```python
from build123d import *

# Parameters (mm, degrees)
EXTRUDE_1_DEPTH     = 17.6
FILLET_2_R          = 2
FILLET_3_R          = 8
SKETCH_2_R          = 10
CUT_EXTRUDE_1_DEPTH = 2


with BuildPart() as part:
    # 草圖1 → 填料-伸長1 (new body)
    with BuildSketch(Plane(origin=(0, 0, 0), x_dir=(1, 0, 0), z_dir=(0, 1, 0))):
        with BuildLine():
            Line((-20.05, 15.65), (20.05, 15.65))
            ThreePointArc((20.05, 15.65), (35.7, 0), (20.05, -15.65))
            Line((20.05, -15.65), (-20.05, -15.65))
            ThreePointArc((-20.05, -15.65), (-35.7, 0), (-20.05, 15.65))
        make_face()
    extrude(amount=EXTRUDE_1_DEPTH)

    # 圓角2
    fillet_2_edges = [part.edges().sort_by_distance(p)[0] for p in [
        (35.7, 17.6, 0),
        (0, 17.6, -15.65),
        (-35.7, 17.6, 0),
        (0, 17.6, 15.65),
    ]]
    fillet(fillet_2_edges, radius=FILLET_2_R)

    # 圓角3
    fillet_3_edges = [part.edges().sort_by_distance(p)[0] for p in [
        (0, 0, -15.65),
        (35.7, 0, 0),
        (0, 0, 15.65),
        (-35.7, 0, 0),
    ]]
    fillet(fillet_3_edges, radius=FILLET_3_R)

    # 草圖2 → 除料-伸長1 (cut)
    with BuildSketch(Plane(origin=(0, 17.6, 0), x_dir=(1, 0, 0), z_dir=(0, 1, 0))):
        with Locations(Location((-11.455400627, 0, 0), (0, 0, 270))):
            Circle(SKETCH_2_R)
    extrude(amount=-CUT_EXTRUDE_1_DEPTH, mode=Mode.SUBTRACT)


solid = part.part
```
Geometry check sheet. Reference: the model listing, model coordinates, mm. Round coordinates to 2 decimals unless told otherwise and drop trailing zeros. Order: outer loops, then holes, each group sorted by start corner. A loop starts at its lowest first (then second) coordinate and runs counter-clockwise, first axis right, second up. Notation, with made-up numbers: M 65.5,-12.5 L 115.5,-12.5 A20 ccw 115.5,2.5 Z; hole C -30,-9.75 d10. An arc over 180 degrees is marked long. Write item = value, one per line.
Q1. Section check A-A (x = 11.5). Enter the section's corners in (y, z).
Answer block:
outline = M 0,-7.65 A8 ccw 8,-15.65 L 15.6,-15.65 A2 ccw 17.6,-13.65 L 17.6,13.65 A2 ccw 15.6,15.65 L 8,15.65 A8 ccw 0,7.65 Z
Q2. Section check C-C (x = -9). Enter the section's corners in (y, z), plus the area to 3 significant figures.
Answer block:
outline = M 0,-7.65 A8 ccw 8,-15.65 L 15.6,-15.65 A2 ccw 17.6,-13.65 L 17.6,-9.69 L 15.6,-9.69 L 15.6,9.69 L 17.6,9.69 L 17.6,13.65 A2 ccw 15.6,15.65 L 8,15.65 A8 ccw 0,7.65 Z
area = 483 mm^2
Q3. Section check B-B (y = 8.75). Enter the section's corners in (x, z), plus the area to 3 significant figures.
Answer block:
outline = M -20.05,-15.65 L 20.05,-15.65 A15.65 ccw 20.05,15.65 L -20.05,15.65 A15.65 ccw Z
area = 2,020 mm^2
Q4. Depth check by flat-ended pin: pin 1 Ø4 at (y, z) = (9.5, 4.5) entering from -X; pin 2 Ø5 at (x, y) = (8.5, 4) entering from +Z; pin 3 Ø2 at (y, z) = (4.5, 5.5) entering from -X. Enter the tip coordinate at first touch or a pass-through.
Answer block:
pin_1 = -35.5
pin_2 = 15.51
pin_3 = -34.42
Q5. Release check for a two-part mould opening along X. For faces 1 (the flat face through (-11, 15.6, 0)), 2 (the cylindrical face through (-21.218, 16.614, -2.168)), 3 (the cylindrical face through (35.696, 11.747, -0.344)), 4 (the cylindrical face through (-0.28, 17, 15.08)) record: released by +X, released by -X, zero draft, split by the parting line, or undercut.
Answer block:
face_1 = undercut
face_2 = undercut
face_3 = released by +X
face_4 = zero draft
Q6. Scan lines: line 1 (X direction, y = 17.1, z = 0); line 2 (X direction, y = 16.75, z = 0); line 3 (Y direction, x = -20, z = -2). Record each from-to range of solid material in increasing order.
Answer block:
line_1 = -35.02 to -21.46, -1.46 to 35.02
line_2 = -35.34 to -21.46, -1.46 to 35.34
line_3 = 0 to 15.6
